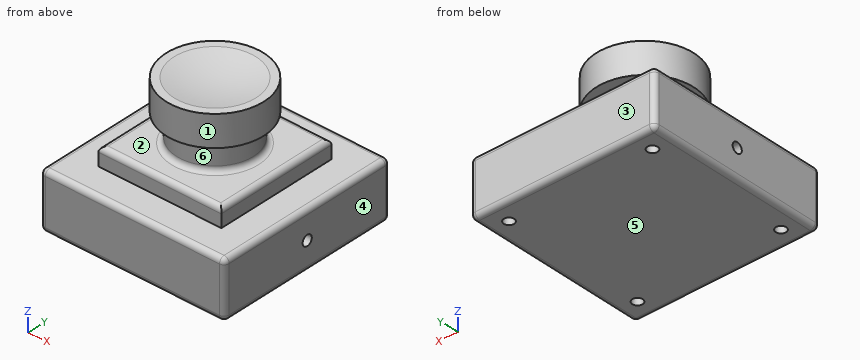
from build123d import *

# Parameters (mm, degrees)
SKETCH_1_W          = 36
SKETCH_1_H          = 36
EXTRUDE_1_DEPTH     = 11
SKETCH_2_W          = 24
SKETCH_2_H          = 24
EXTRUDE_2_DEPTH     = 3.5
SKETCH_3_R          = 7.5
EXTRUDE_3_DEPTH     = 5.5
SKETCH_4_R          = 9.5
EXTRUDE_4_DEPTH     = 6
FILLET_1_R          = 1
SKETCH_6_R          = 1
CUT_EXTRUDE_1_DEPTH = 5
SKETCH_7_R          = 1
CUT_EXTRUDE_2_DEPTH = 5


with BuildPart() as part:
    # 草图1 → 凸台-拉伸1 (new body)
    with BuildSketch(Plane.XY):
        Rectangle(SKETCH_1_W, SKETCH_1_H)
    extrude(amount=EXTRUDE_1_DEPTH)

    # 草图2 → 凸台-拉伸2 (add)
    with BuildSketch(Plane.XY.offset(11)):
        Rectangle(SKETCH_2_W, SKETCH_2_H)
    extrude(amount=EXTRUDE_2_DEPTH)

    # 草图3 → 凸台-拉伸3 (add)
    with BuildSketch(Plane.XY.offset(14.5)):
        Circle(SKETCH_3_R)
    extrude(amount=EXTRUDE_3_DEPTH)

    # 草图4 → 凸台-拉伸4 (add)
    with BuildSketch(Plane.XY.offset(20)):
        Circle(SKETCH_4_R)
    extrude(amount=EXTRUDE_4_DEPTH)

    # 草图5 → 切除-旋转1 (revolve, cut)
    with BuildSketch(Plane(origin=(0, 0, 0), x_dir=(1, 0, 0), z_dir=(0, 1, 0))):
        with BuildLine():
            Line((0, -24.91366459), (0, -26))
            Line((0, -26), (8, -26))
            ThreePointArc((8, -26), (4.036710437, -25.186488995), (0, -24.91366459))
        make_face()
    revolve(axis=Axis((0, 0, 24.353707744), (0, 0, 1)), mode=Mode.SUBTRACT)

    # 圆角1
    fillet_1_edges = [part.edges().sort_by_distance(p)[0] for p in [
        (-18, 0, 11),
        (0, -18, 11),
        (-12, 0, 14.5),
        (0, -12, 14.5),
        (12, 0, 14.5),
        (0, 12, 14.5),
        (-7.5, 0, 14.5),
        (18, 0, 11),
        (0, -18, 0),
        (-18, 0, 0),
        (0, 18, 0),
        (18, 0, 0),
        (18, -18, 5.5),
        (-18, -18, 5.5),
        (-18, 18, 5.5),
        (18, 18, 5.5),
        (0, 18, 11),
    ]]
    fillet(fillet_1_edges, radius=FILLET_1_R)

    # 草图6 → 切除-拉伸1 (cut)
    with BuildSketch(Plane(origin=(18, 0, 0), x_dir=(0, 0, -1), z_dir=(1, 0, 0))):
        with Locations((-5.5, 0)):
            Circle(SKETCH_6_R)
    cut_extrude_1 = extrude(amount=-CUT_EXTRUDE_1_DEPTH, mode=Mode.SUBTRACT)

    # 镜向1: 切除-拉伸1 across plane
    add(cut_extrude_1.mirror(Plane(origin=(0, 0, 0), x_dir=(0, 0, 1), z_dir=(1, 0, 0))), mode=Mode.SUBTRACT)

    # 草图7 → 切除-拉伸2 (cut)
    with BuildSketch(Plane(origin=(0, 0, 0), x_dir=(-1, 0, 0), z_dir=(0, 0, -1))):
        with Locations((-14, 14)):
            Circle(SKETCH_7_R)
        with Locations(Location((-14, -14, 0), (0, 0, 180))):
            Circle(SKETCH_7_R)
        with Locations((14, -14)):
            Circle(SKETCH_7_R)
        with Locations(Location((14, 14, 0), (0, 0, 180))):
            Circle(SKETCH_7_R)
    extrude(amount=-CUT_EXTRUDE_2_DEPTH, mode=Mode.SUBTRACT)


solid = part.part
Can you work these out from the model? Positions are in its coordinate system, mm. Face numbers are marked on the shaded views. A direction names the side the tool comes from. Coordinates: 2 decimals unless noted, no trailing zeros. Write each loop counter-clockwise with the first axis right and the second up, starting at its lowest first coordinate (ties: lowest second). Pieces come first, ordered by that corner, then holes. Notation, with made-up numbers: (56, 79) - (109, 79) arc R35 ccw to (109, 116) - close; hole circle Ø1 at (-11.5, 26.5). An arc over 180 degrees is marked (long way). Return JSON: item names as keys, results as strings. Group by question number.
Item 1: Please list where these lines run through material, in increasing order: probe 1 along Y at (x, z) = (-14, 3.2); probe 2 along Z at (x, y) = (4, 8.5); probe 3 along X at (y, z) = (-14.5, 3.25).
Item 2: I'm going to push flat-ended pins straight in: pin 1 Ø1.6 at (y, z) = (0, 5.5) entering from -X; pin 2 Ø1.2 at (y, z) = (-5, 12.5) entering from +X; pin 3 Ø1.2 at (x, z) = (1.5, 12.5) entering from -Y. Where does each tip first touch, or does it pass through?
Item 3: If we section it at B-B (x = 14): Write out the boundary of the cut face in (y, z), then the cut area to 3 significant figures.
Item 4: We'd pull the mould along Z, two halves only. Please class the marked faces 4, 5 and 6: pulls with the +Z half, pulls with the -Z half, needs draft (parallel to the pull), parting line crosses it, or undercut.
Item 5: If we section it at A-A (x = -12.5): Write out the boundary of the cut face in (y, z), then the cut area to 3 significant figures.
Item 6: Which directions (+Z, -Z, +X, -X, +Y, -Y) give clear straight access to the entire face, cutting with the end or side of a thin tool? Please do the marked faces 1, 2 and 3.
Item 7: If we section it at D-D (z = 5.5): Write out the boundary of the cut face in (x, y).
Item 8: If we section it at C-C (y = 14): Write out the boundary of the cut face in (x, z), then the cut area to 3 significant figures.
Return value:
{
 "1": {"probe 1": "y = -18 to -15, -13 to 13, 15 to 18", "probe 2": "z = 0 to 14.5, 20 to 26", "probe 3": "x = -18 to -14.87, -13.13 to 13.13, 14.87 to 18"},
 "2": {"pin 1": "stops at x = -13", "pin 2": "stops at x = 12", "pin 3": "stops at y = -12"},
 "3": {"outline": "(-18, 1) arc R1 ccw to (-17, 0) - (-15, 0) - (-15, 5) - (-13, 5) - (-13, 0) - (13, 0) - (13, 5) - (15, 5) - (15, 0) - (17, 0) arc R1 ccw to (18, 1) - (18, 10) arc R1 ccw to (17, 11) - (-17, 11) arc R1 ccw to (-18, 10) - close; hole circle Ø2 at (0, 5.5)", "area": "372 mm^2"},
 "4": {"face 4": "needs draft", "face 5": "pulls with the -Z half", "face 6": "undercut"},
 "5": {"outline": "(-18, 1) arc R1 ccw to (-17, 0) - (17, 0) arc R1 ccw to (18, 1) - (18, 10) arc R1 ccw to (17, 11) - (-17, 11) arc R1 ccw to (-18, 10) - close", "area": "395 mm^2"},
 "6": {"face 1": "+Z", "face 2": "none", "face 3": "+Z, -Z, +X, -X, +Y"},
 "7": {"outline": "(-18, -17) arc R1 ccw to (-17, -18) - (17, -18) arc R1 ccw to (18, -17) - (18, -1) - (13, -1) - (13, 1) - (18, 1) - (18, 17) arc R1 ccw to (17, 18) - (-17, 18) arc R1 ccw to (-18, 17) - (-18, 1) - (-13, 1) - (-13, -1) - (-18, -1) - close"},
 "8": {"outline": "(-18, 1) arc R1 ccw to (-17, 0) - (-15, 0) - (-15, 5) - (-13, 5) - (-13, 0) - (13, 0) - (13, 5) - (15, 5) - (15, 0) - (17, 0) arc R1 ccw to (18, 1) - (18, 10) arc R1 ccw to (17, 11) - (-17, 11) arc R1 ccw to (-18, 10) - close", "area": "375 mm^2"}
}
